Here's the drawing with two shaded views (mm, measured from the low corner). I have some questions. Give positions to 0.01 mm unless a question says otherwise; leave off trailing zeros. Order: outer loops, then holes, each group sorted by start corner. A loop starts at its lowest first (then second) coordinate and runs counter-clockwise, first axis right, second up. Notation, with made-up numbers: (-25, 79.5) - (-15, 79.5) arc R25 cw to (-15, 97.5) - close; hole circle Ø2 at (4.5, 21). An arc over 180 degrees is marked (long way). Use one line per item in the form item = value. Start each with the question number.
1) Suppose I cut it at A-A, the plane z = 7. Write out the boundary of the cut face in (x, y).
2) Suppose I cut it at C-C, the plane x = 2.25. Write out the boundary of the cut face in (y, z), and give its area (3 significant figures).
3) Please list where these lines run through material, in increasing order: probe 1 along Y at (x, z) = (5.7, 7); probe 2 along Z at (x, y) = (6.45, 615); probe 3 along X at (y, z) = (397.5, 7.5).
4) For pin 1 (4 mm diameter, centred on y = 611.5, z = 4, fed in from -X); pin 2 (2 mm diameter, centred on x = 5.5, z = 8.5, fed in from -Y); pin 3 (1 mm diameter, centred on x = 11.5, y = 356, fed in from -Z); pin 4 (4 mm diameter, centred on x = 11, y = 345, fed in from -Z), each with a flat end and sliding along its axis, tell me the tip position at first contact or that it passes through.
5) Suppose I cut it at B-B, the plane y = 355. Write out the boundary of the cut face in (x, z).
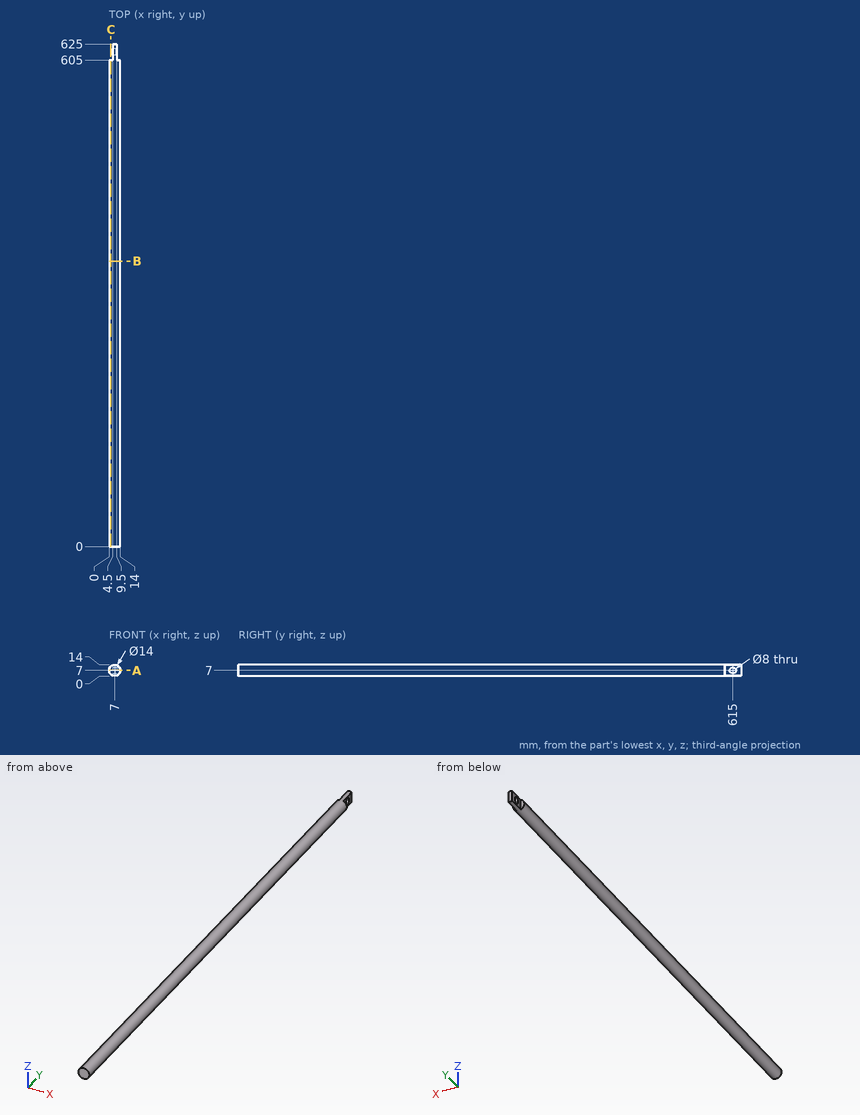
Result sheet:
q1.outline = (0, 0) - (14, 0) - (14, 605) - (9.5, 605) - (9.5, 611) - (4.5, 611) - (4.5, 605) - (0, 605) - close; (4.5, 619) - (9.5, 619) - (9.5, 625) - (4.5, 625) - close
q2.outline = (0, 1.86) - (605, 1.86) - (605, 12.14) - (0, 12.14) - close
q2.area = 6,220 mm²
q3.probe_1 = 0 to 611, 619 to 625
q3.probe_2 = 0.02 to 3, 11 to 13.98
q3.probe_3 = 0.02 to 13.98
q4.pin_1 = 4.5
q4.pin_2 = 0
q4.pin_3 = 1.26
q4.pin_4 = 0.29
q5.outline = circle Ø14 at (7, 7)
